Build history of the part. All positions in model axes, mm. Face numbers are marked on the shaded views. A direction names the side the tool comes from. Round coordinates to 2 decimals unless told otherwise and drop trailing zeros. Write each loop counter-clockwise with the first axis right and the second up, starting at its lowest first coordinate (ties: lowest second). Pieces come first, ordered by that corner, then holes. Notation, with made-up numbers: (17.25, 45.25) - (62.25, 45.25) arc R20 cw to (62.25, 73.25) - close; hole circle Ø1 at (38, 88). An arc over 180 degrees is marked (long way). Write each question's results on one line, items separated by ' | '.
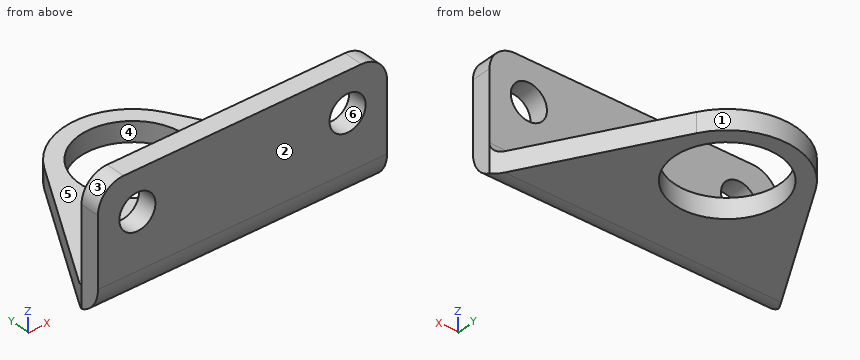
from build123d import *

# Parameters (mm, degrees)
EXTRUDE_START                   = -22
EXTRUDE_1_DEPTH                 = 44
CUT_EXTRUDE_1_DEPTH             = 10
CUT_EXTRUDE_1_DIRECTION_2_REACH = 42.869
SKETCH_6_R                      = 8
CUT_EXTRUDE_2_DEPTH             = 41.868692174
SKETCH_7_R                      = 2.75
CUT_EXTRUDE_3_DEPTH             = 41.015621949
FILLET_1_R                      = 3.9


with BuildPart() as part:
    # 草图4 → 凸台-拉伸1 (new body)
    with BuildSketch(Plane(origin=(0, 0, 0), x_dir=(0, 0, -1), z_dir=(1, 0, 0)).offset(EXTRUDE_START)):
        with BuildLine():
            Line((-19, 0), (-4.625, 0))
            ThreePointArc((-4.625, 0), (-1.354631137, 1.354631137), (0, 4.625))
            Line((0, 4.625), (0, 30.5))
            Line((0, 30.5), (-3, 30.5))
            Line((-3, 30.5), (-3, 4.625))
            ThreePointArc((-3, 4.625), (-3.475951481, 3.475951481), (-4.625, 3))
            Line((-4.625, 3), (-19, 3))
            Line((-19, 3), (-19, 0))
        make_face()
    extrude(amount=EXTRUDE_1_DEPTH)

    # 草图5 → 切除-拉伸1 (cut)
    with BuildSketch(Plane.XY.offset(3)):
        with BuildLine():
            Line((-9.082524892, 25.268561625), (-22, 3))
            Line((-22, 3), (-22, 31.5))
            Line((-22, 31.5), (22, 31.5))
            Line((22, 31.5), (22, 3))
            Line((22, 3), (9.082524892, 25.268561625))
            ThreePointArc((9.082524892, 25.268561625), (0, 30.5), (-9.082524892, 25.268561625))
        make_face()
    extrude(amount=-CUT_EXTRUDE_1_DEPTH, mode=Mode.SUBTRACT)

    # 切除-拉伸1 direction 2: up to this face of the body (flat: up to its plane)
    cut_extrude_1_direction_2_end = Plane(part.part.faces().sort_by_distance((0, 1.5, 19))[0])
    # 草图5 → 切除-拉伸1 direction 2 (cut, up to the picked face)
    with BuildSketch(Plane.XY.offset(3), mode=Mode.PRIVATE) as cut_extrude_1_direction_2_sk1:
        with BuildLine():
            Line((-9.082524892, 25.268561625), (-22, 3))
            Line((-22, 3), (-22, 31.5))
            Line((-22, 31.5), (22, 31.5))
            Line((22, 31.5), (22, 3))
            Line((22, 3), (9.082524892, 25.268561625))
            ThreePointArc((9.082524892, 25.268561625), (0, 30.5), (-9.082524892, 25.268561625))
        make_face()
    cut_extrude_1_direction_2_tool1 = split(extrude(cut_extrude_1_direction_2_sk1.sketch, amount=CUT_EXTRUDE_1_DIRECTION_2_REACH, mode=Mode.PRIVATE), bisect_by=cut_extrude_1_direction_2_end, keep=Keep.BOTH, mode=Mode.PRIVATE)
    add(cut_extrude_1_direction_2_tool1.solids().sort_by(Axis((-15.994729, 14.397326, 3), (0, 0, 1)))[0], mode=Mode.SUBTRACT)

    # 草图6 → 切除-拉伸2 (cut, through all)
    with BuildSketch(Plane.XY.offset(3)):
        with Locations((0, 20)):
            Circle(SKETCH_6_R)
    extrude(amount=-CUT_EXTRUDE_2_DEPTH, mode=Mode.SUBTRACT)

    # 草图7 → 切除-拉伸3 (cut, through all)
    with BuildSketch(Plane(origin=(0, 3, 0), x_dir=(1, 0, 0), z_dir=(0, 1, 0))):
        with Locations(Location((16, -13, 0), (0, 0, 270))):
            Circle(SKETCH_7_R)
        with Locations(Location((-16, -13, 0), (0, 0, 90))):
            Circle(SKETCH_7_R)
    extrude(amount=-CUT_EXTRUDE_3_DEPTH, mode=Mode.SUBTRACT)

    # 圆角1
    fillet_1_edges = [part.edges().sort_by_distance(p)[0] for p in [
        (-22, 1.5, 19),
        (22, 1.5, 19),
    ]]
    fillet(fillet_1_edges, radius=FILLET_1_R)


solid = part.part
(1) Slice it at B-B, the plane x = 0. Write the cut outline in (y, z) (3 decimals).
Worked answers:
outline: (0, 4.625) arc R4.625 ccw to (4.625, 0) - (12, 0) - (12, 3) - (4.625, 3) arc R1.625 cw to (3, 4.625) - (3, 19) - (0, 19) - close; (28, 0) - (30.5, 0) - (30.5, 3) - (28, 3) - close
(2) Slice it at C-C, the plane y = 13.5. Write the cut outline in (x, z), and give its area (3 significant figures).
Worked answers:
outline: (-15.91, 0) - (-4.66, 0) - (-4.66, 3) - (-15.91, 3) - close; (4.66, 0) - (15.91, 0) - (15.91, 3) - (4.66, 3) - close | area: 67.5 mm2
(3) Flat gauge pins, fed straight in: pin 1 Ø2 at (y, z) = (19, 3) entering from -X; pin 2 Ø7 at (x, z) = (3, 11.5) entering from +Y; pin 3 Ø4 at (x, y) = (10.5, 24.5) entering from +Z. Where does each tip first touch, or does it go through?
Worked answers:
pin 1: stops at x = -13.3 | pin 2: stops at y = 3 | pin 3: stops at z = 3
(4) Drill centre lines: probe 1 along X at (y, z) = (1.45, 13); probe 2 along Y at (x, z) = (6.5, 12.25); probe 3 along Y at (x, z) = (0, 2.2). Where is each one in solid material? Low to high. Write a range as [from, to].
Worked answers:
probe 1: x = [-22, -18.75], [-13.25, 13.25], [18.75, 22] | probe 2: y = [0, 3] | probe 3: y = [0.69, 12], [28, 30.5]
(5) Two-plate mould, pull along Y, no slides. Class the marked faces 1, 2, 3 and 4: released by +Y, released by -Y, zero draft, split by the parting line, or undercut.
Worked answers:
face 1: released by +Y | face 2: released by -Y | face 3: zero draft | face 4: undercut
(6) Slice it at D-D, the plane y = 2. Write the cut outline in (x, z), and give its area (3 significant figures).
Worked answers:
outline: (-22, 0.82) - (22, 0.82) - (22, 15.1) arc R3.9 ccw to (18.1, 19) - (-18.1, 19) arc R3.9 ccw to (-22, 15.1) - close; hole circle Ø5.5 at (-16, 13); hole circle Ø5.5 at (16, 13) | area: 746 mm2
(7) Slice it at A-A, the plane z = 13. Write the cut outline in (x, y).
Worked answers:
outline: (-22, 0) - (-18.75, 0) - (-18.75, 3) - (-22, 3) - close; (-13.25, 0) - (13.25, 0) - (13.25, 3) - (-13.25, 3) - close; (18.75, 0) - (22, 0) - (22, 3) - (18.75, 3) - close
(8) Tool access for the marked faces 5 and 6: list every direction of +Z, -Z, +X, -X, +Y, -Y with a clear straight run to the whole face (end or side of a thin tool).
Worked answers:
face 5: +Z, +X, -X, +Y | face 6: +Y, -Y
